from build123d import *

# Parameters (mm, degrees)
SKETCH1_R           = 3.81
BOSS_EXTRUDE1_DEPTH = 139.7
SKETCH2_R           = 6.35
BOSS_EXTRUDE2_DEPTH = 2.54
BOSS_EXTRUDE3_START = 2.54
SKETCH3_R           = 6.35
BOSS_EXTRUDE3_DEPTH = 2.54


with BuildPart() as part:
    # Sketch1 → Boss-Extrude1 (new body)
    with BuildSketch(Plane(origin=(0, 0, 0), x_dir=(0, 0, -1), z_dir=(1, 0, 0))):
        Circle(SKETCH1_R)
    extrude(amount=BOSS_EXTRUDE1_DEPTH)

    # Sketch2 → Boss-Extrude2 (add)
    with BuildSketch(Plane(origin=(139.7, 0, 0), x_dir=(0, 0, -1), z_dir=(1, 0, 0))):
        Circle(SKETCH2_R)
    extrude(amount=BOSS_EXTRUDE2_DEPTH)

    # Sketch3 → Boss-Extrude3 (add)
    with BuildSketch(Plane.ZY.offset(BOSS_EXTRUDE3_START)):
        with Locations(Location((0, 0, 0), (0, 0, 180))):
            Circle(SKETCH3_R)
    extrude(amount=-BOSS_EXTRUDE3_DEPTH)


solid = part.part
Here's how the part is built. I have some questions about the finished solid (model axes, mm). A direction names the side the tool comes from. Coordinates: 2 decimals unless noted, no trailing zeros. Loops run counter-clockwise (first coordinate to the right, second up) from the corner with the lowest first, then second, coordinate; pieces in that order, holes last.
1. For P1, Ø3, axis at x = 15.5, y = -4, coming from the +Z side; P2, Ø1.5, axis at y = -5, z = -4, coming from the +X side; P3, Ø5, axis at x = 61, z = 2.5, coming from the +Y side; P4, Ø6, axis at x = 20, z = -1, coming from the -Y side, each with a flat end and sliding along its axis, tell me the tip position at first contact or that it passes through.
2. If we mould it in two halves opening along X, with no side actions, what happens to faces 1 (the flat face through (0, 3, -3)), 2 (the flat face through (142.24, 0, 0)), 3 (the cylindrical face through (140.95, -6.2, 1.38))? For each: pulls with the +X half, pulls with the -X half, needs draft (parallel to the pull), parting line crosses it, or undercut.
3. I need wall thicknesses on L1, parallel to X at y = 4.75, z = 2.75; L2, parallel to Z at x = 59.5, y = 0.25; L3, parallel to Z at x = 77.5, y = -2. Which ranges of each line are inside material? Lowest first, please.
4. For faces 4 (the flat face through (139.7, -3, -3)), 5 (the flat face through (-2.54, 0, 0)), which set-ups out of +Z, -Z, +X, -X, +Y, -Y let a thin tool reach every point of the face, with its end or its side?
5. Imagine slicing it at C-C, the plane x = 111.5. Please give me the cut outline in (y, z), and give its area (3 significant figures).
6. Imagine slicing it at A-A, the plane z = 0. Please give me the cut outline in (x, y), and give its area (3 significant figures).
Taken from the geometry:
1. P1: stops at z = 2.88
1. P2: stops at x = 142.24
1. P3: stops at y = 3.81
1. P4: stops at y = -3.81
2. face 1: undercut
2. face 2: pulls with the +X half
2. face 3: needs draft
3. L1: x = -2.54 to 0, 139.7 to 142.24
3. L2: z = -3.8 to 3.8
3. L3: z = -3.24 to 3.24
4. face 4: none
4. face 5: +Z, -Z, -X, +Y, -Y
5. outline: circle Ø7.62 at (0, 0)
5. area: 45.6 mm2
6. outline: (-2.54, -6.35) - (0, -6.35) - (0, -3.81) - (139.7, -3.81) - (139.7, -6.35) - (142.24, -6.35) - (142.24, 6.35) - (139.7, 6.35) - (139.7, 3.81) - (0, 3.81) - (0, 6.35) - (-2.54, 6.35) - close
6. area: 1,130 mm2
